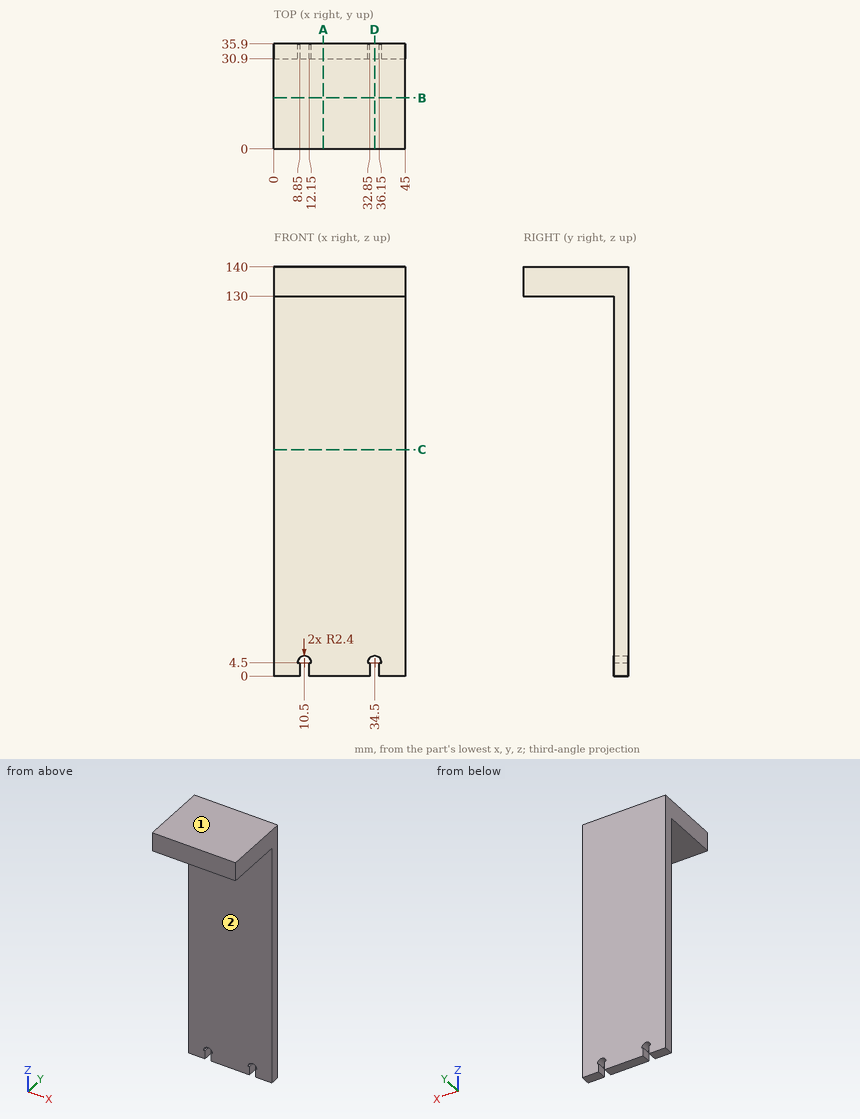
Geometry check sheet. Reference: drawing and pictorial views, mm from the part's lowest x, y, z. A direction names the side the tool comes from. Give positions to 0.01 mm unless a question says otherwise; leave off trailing zeros. Write each loop counter-clockwise with the first axis right and the second up, starting at its lowest first coordinate (ties: lowest second). Pieces come first, ordered by that corner, then holes. Notation, with made-up numbers: M 17,11 L 37,11 A17 ccw 37,28 Z; hole C 58,-8.75 d5. An arc over 180 degrees is marked long. Use CSV: the item, a comma, the result in double quotes.
1) Cross-section at C-C (z = 77.5). Enter the section's corners in (x, y), plus the area to 3 significant figures.
Final values:
outline,"M 0,30.9 L 45,30.9 L 45,35.9 L 0,35.9 Z"
area,"225 mm²"
2) Cross-section at D-D (x = 34.5). Enter the section's corners in (y, z), plus the area to 4 significant figures.
Final values:
outline,"M 0,130 L 30.9,130 L 30.9,6.9 L 35.9,6.9 L 35.9,140 L 0,140 Z"
area,"974.5 mm²"
3) Access from +Z, -Z, +X, -X, +Y, -Y to the whole of each face (thin tool, end or side, straight path). Record for the marked faces 1 and 2.
Final values:
face 1,"+Z, +X, -X, +Y, -Y"
face 2,"-Z, +X, -X, -Y"
4) Go/stop test with flat-tipped pins: pin 1 Ø8 at (x, z) = (19.5, 29.5) entering from -Y; pin 2 Ø1.5 at (x, y) = (32.5, 29) entering from -Z. Record where each tip stops, or that it passes through.
Final values:
pin 1,"y = 30.9"
pin 2,"z = 130"
5) Material ranges on line 1 along Z through (x, y) = (40.5, 11); line 2 along Y through (x, z) = (16.5, 82.5), recorded low to high.
Final values:
line 1,"130 to 140"
line 2,"30.9 to 35.9"
6) Cross-section at B-B (y = 17.5). Enter the section's corners in (x, z), plus the area to 3 significant figures.
Final values:
outline,"M 0,130 L 45,130 L 45,140 L 0,140 Z"
area,"450 mm²"
7) Cross-section at A-A (x = 17). Enter the section's corners in (y, z), plus the area to 3 significant figures.
Final values:
outline,"M 0,130 L 30.9,130 L 30.9,0 L 35.9,0 L 35.9,140 L 0,140 Z"
area,"1,010 mm²"
